```python
from build123d import *

# Parameters (mm, degrees)
F0_W      = 40
F0_H      = 69.2
F0_W_2    = 36
F0_H_2    = 65.2
F1_DEPTH  = 2
F2_W      = 20
F2_H      = 2
F3_DEPTH  = 2
F4_W      = 40
F4_H      = 69.2
F5_DEPTH  = 2
F6_R      = 7.99999
F7_R      = 9
F8_R      = 2
F10_DEPTH = 2
F11_R     = 5


# Not quite as in the source:
# - a fillet or chamfer is up to 0.001 mm smaller than in the source, because OpenCascade refuses the exact size


with BuildPart() as f1:
    # F0 (on Top) → F1 (new body)
    with BuildSketch(Plane.XY):
        with Locations((0, 0.4)):
            Rectangle(F0_W, F0_H)
        with Locations((0, 0.4)):
            Rectangle(F0_W_2, F0_H_2, mode=Mode.SUBTRACT)
    extrude(amount=F1_DEPTH)

    # F2 (on Top) → F3 (join, symmetric)
    with BuildSketch(Plane.XY):
        with Locations((0, -31.35)):
            Rectangle(F2_W, F2_H)
        with Locations((0, 32.15)):
            Rectangle(F2_W, F2_H)
    extrude(amount=F3_DEPTH, both=True)

    # F4 (on face) → F5 (join)
    with BuildSketch(Plane.XY.offset(2)):
        with Locations((0, 0.4)):
            Rectangle(F4_W, F4_H)
        with BuildLine():
            ThreePointArc((6, 10.7552776188), (0, 8.7552776188), (-6, 10.7552776188))
            Line((-6, 10.7552776188), (6, 10.7552776188))
        make_face(mode=Mode.SUBTRACT)
        with BuildLine():
            ThreePointArc((-8, 12.7552776188), (-8.6406368723, 13.721452588), (-9.1651513899, 14.7552776188))
            Line((-9.1651513899, 14.7552776188), (9.1651513899, 14.7552776188))
            ThreePointArc((9.1651513899, 14.7552776188), (8.6406368723, 13.721452588), (8, 12.7552776188))
            Line((8, 12.7552776188), (-8, 12.7552776188))
        make_face(mode=Mode.SUBTRACT)
        with BuildLine():
            Line((9.7979589711, 16.7552776188), (-9.7979589711, 16.7552776188))
            ThreePointArc((-9.7979589711, 16.7552776188), (-10, 18.7552776188), (-9.7979589711, 20.7552776188))
            Line((-9.7979589711, 20.7552776188), (9.7979589711, 20.7552776188))
            ThreePointArc((9.7979589711, 20.7552776188), (10, 18.7552776188), (9.7979589711, 16.7552776188))
        make_face(mode=Mode.SUBTRACT)
        with BuildLine():
            Line((9.1651513899, 22.7552776188), (-9.1651513899, 22.7552776188))
            ThreePointArc((-9.1651513899, 22.7552776188), (-8.6406368723, 23.7891026495), (-8, 24.7552776188))
            Line((-8, 24.7552776188), (8, 24.7552776188))
            ThreePointArc((8, 24.7552776188), (8.6406368723, 23.7891026495), (9.1651513899, 22.7552776188))
        make_face(mode=Mode.SUBTRACT)
        with BuildLine():
            Line((6, 26.7552776188), (-6, 26.7552776188))
            ThreePointArc((-6, 26.7552776188), (0, 28.7552776188), (6, 26.7552776188))
        make_face(mode=Mode.SUBTRACT)
    extrude(amount=F5_DEPTH)

    # F6 (radius 8 in the source; OpenCascade refuses exactly that, so slightly less here)
    f6_edges = [f1.edges().sort_by_distance(p)[0] for p in [
        (18, 33, 1),
        (-18, 33, 1),
        (18, -32.2, 1),
        (-18, -32.2, 1),
    ]]
    fillet(f6_edges, radius=F6_R)

    # F7
    f7_edges = [f1.edges().sort_by_distance(p)[0] for p in [
        (-20, -34.2, 2),
        (-20, 35, 2),
        (20, 35, 2),
        (20, -34.2, 2),
    ]]
    fillet(f7_edges, radius=F7_R)

    # F8
    f8_edges = [f1.edges().sort_by_distance(p)[0] for p in [
        (20, 0.4, 4),
    ]]
    fillet(f8_edges, radius=F8_R)

    # F9 (on face) → F10 (join)
    with BuildSketch(Plane(origin=(0, 0, 0), x_dir=(1, 0, 0), z_dir=(0, 0, -1))):
        with BuildLine():
            Line((3, 34.2), (5, 34.2))
            ThreePointArc((5, 34.2), (0, 39.2), (-5, 34.2))
            Line((-5, 34.2), (-3, 34.2))
            ThreePointArc((-3, 34.2), (0, 37.2), (3, 34.2))
        make_face()
    extrude(amount=-F10_DEPTH)

    # F11
    f11_edges = [f1.edges().sort_by_distance(p)[0] for p in [
        (-5, -34.2, 1),
        (5, -34.2, 1),
    ]]
    fillet(f11_edges, radius=F11_R)


solid = f1.part
```
CAD build for the part. Positions are in the model's coordinates, mm. A direction names the side the tool comes from. Round coordinates to 2 decimals unless told otherwise and drop trailing zeros. Write each loop counter-clockwise with the first axis right and the second up, starting at its lowest first coordinate (ties: lowest second). Pieces come first, ordered by that corner, then holes. Notation, with made-up numbers: (3.25, 87.5) - (60.25, 87.5) arc R32 cw to (60.25, 114.5) - close; hole circle Ø5 at (0.25, -30.75). An arc over 180 degrees is marked (long way). Return JSON: item names as keys, results as strings. Group by question number.
Item 1: Band-saw the part on B-B on y = 19. List the corners of the cut face in (x, z), plus the area to 3 significant figures.
Item 2: Mould opens along X. For faces 1 (the face through (-0.1, -37.2, 1)), 2 (the face through (17.294, 32.434, 0.986)), 3 (the face through (0, 35, 1)) say: +X half, -X half, draft (parallel to the pull), parting line (faces both ways), or undercut.
Item 3: 3-axis set-ups, long thin cutter, end or side, ignore diameter. For faces 4 (the face through (10, 18.8, 3)), 5 (the face through (10, -34.2, 1)), 6 (the face through (10, 32, 0)): which of +Z, -Z, +X, -X, +Y, -Y reach the whole face in a straight line?
Item 4: Band-saw the part on A-A on z = 1.15. State how many separate pieces and enclosed holes the cut face has, plus the area to 3 significant figures.
Item 5: Flat gauge pins, fed straight in: pin 1 Ø2 at (y, z) = (-31.5, 0.5) entering from -X; pin 2 Ø3 at (x, z) = (-8.5, 1) entering from -Y; pin 3 Ø0.6 at (x, z) = (-1.5, 3.5) entering from -Y. Where does each tip first touch, or does it go through?
Item 6: Band-saw the part on D-D on y = -6. List the corners of the cut face in (x, z).
Item 7: Probe probe 1 along X at (y, z) = (25, 1.85); probe 2 along Y at (x, z) = (6, -1.4); probe 3 along Z at (x, y) = (-8, -17). List the from-to ranges inside material, lowest first.
Resolved:
{
 "1": {"outline": "(-20, 0) - (-18, 0) - (-18, 2) - (-10, 2) - (-10, 4) - (-18, 4) arc R2 ccw to (-20, 2) - close; (10, 2) - (18, 2) - (18, 0) - (20, 0) - (20, 2) arc R2 ccw to (18, 4) - (10, 4) - close", "area": "46.3 mm²"},
 "2": {"face 1": "undercut", "face 2": "+X half", "face 3": "draft"},
 "3": {"face 4": "+Z, -Z", "face 5": "+Z, -Z, +X, -Y", "face 6": "-Z"},
 "4": {"separate pieces": "1", "enclosed holes": "2", "area": "509 mm²"},
 "5": {"pin 1": "stops at x = -18.27", "pin 2": "stops at y = -34.48", "pin 3": "stops at y = -33.8"},
 "6": {"outline": "(-20, 0) - (-18, 0) - (-18, 2) - (18, 2) - (18, 0) - (20, 0) - (20, 2) arc R2 ccw to (18, 4) - (-18, 4) arc R2 ccw to (-20, 2) - close"},
 "7": {"probe 1": "x = -20 to -18, 18 to 20", "probe 2": "y = -32.35 to -30.35, 31.15 to 33.15", "probe 3": "z = 2 to 4"}
}
